Geometry: final body of the model. Coordinates: model frame, mm. A direction names the side the tool comes from. Coordinates: 2 decimals unless noted, no trailing zeros. Write each loop counter-clockwise with the first axis right and the second up, starting at its lowest first coordinate (ties: lowest second). Pieces come first, ordered by that corner, then holes. Notation, with made-up numbers: (1.25, 10.25) - (23.25, 10.25) arc R36 ccw to (23.25, 49.25) - close; hole circle Ø10 at (28.25, 26). An arc over 180 degrees is marked (long way). Put each result on its own line as item: value.
```python
from build123d import *

# Parameters (mm, degrees)
SKETCH1_W           = 419.1
SKETCH1_H           = 333.375
BOSS_EXTRUDE1_DEPTH = 107.95
SKETCH2_W           = 139.7
SKETCH2_H           = 50.8
CUT_EXTRUDE1_DEPTH  = 108.95
CHAMFER1_SIZE       = 50.8
CHAMFER1_SIZE2      = 13.611818976
FILLET1_R           = 12.7
SKETCH3_W           = 139.7
SKETCH3_H           = 56.403006085
CUT_EXTRUDE2_DEPTH  = 38.1
SKETCH4_W           = 139.7
SKETCH4_H           = 56.128435861
CUT_EXTRUDE3_DEPTH  = 38.1


with BuildPart() as part:
    # Sketch1 → Boss-Extrude1 (new body)
    with BuildSketch(Plane(origin=(0, 0, 0), x_dir=(1, 0, 0), z_dir=(0, 1, 0))):
        Rectangle(SKETCH1_W, SKETCH1_H)
    extrude(amount=BOSS_EXTRUDE1_DEPTH)

    # Sketch2 → Cut-Extrude1 (cut, through all)
    with BuildSketch(Plane(origin=(0, 107.95, 0), x_dir=(1, 0, 0), z_dir=(0, 1, 0))):
        with Locations((0, -115.8875)):
            Rectangle(SKETCH2_W, SKETCH2_H)
        Polygon((-69.85, -166.6875), (-69.85, -157.1625), (-32.169017961, -166.6875), align=None)
        Polygon((32.169017961, -166.6875), (69.85, -166.6875), (69.85, -157.1625), align=None)
    extrude(amount=-CUT_EXTRUDE1_DEPTH, mode=Mode.SUBTRACT)

    # Chamfer1
    chamfer1_edges = [part.edges().sort_by_distance(p)[0] for p in [
        (69.85, 53.975, 141.2875),
        (-69.85, 53.975, 141.2875),
    ]]
    chamfer1_side = [part.faces().sort_by_distance(p)[0] for p in [
        (0, 53.975, 141.2875),
    ]]
    chamfer(chamfer1_edges, length=CHAMFER1_SIZE, length2=CHAMFER1_SIZE2, reference=chamfer1_side[0])

    # Fillet1
    fillet1_edges = [part.edges().sort_by_distance(p)[0] for p in [
        (69.85, 53.975, 90.4875),
        (-69.85, 53.975, 90.4875),
        (-32.169017961, 53.975, 166.6875),
        (32.169017961, 53.975, 166.6875),
        (69.85, 53.975, 127.675681024),
        (-19.05, 53.975, 141.2875),
        (19.05, 53.975, 141.2875),
        (-69.85, 53.975, 127.675681024),
    ]]
    fillet(fillet1_edges, radius=FILLET1_R)

    # Sketch3 → Cut-Extrude2 (cut)
    with BuildSketch(Plane(origin=(0, 107.95, 0), x_dir=(1, 0, 0), z_dir=(0, 1, 0))):
        with Locations((0, -138.485996957)):
            Rectangle(SKETCH3_W, SKETCH3_H)
    extrude(amount=-CUT_EXTRUDE2_DEPTH, mode=Mode.SUBTRACT)

    # Sketch4 → Cut-Extrude3 (cut)
    with BuildSketch(Plane.XZ):
        with Locations((0, 138.623282069)):
            Rectangle(SKETCH4_W, SKETCH4_H)
    extrude(amount=-CUT_EXTRUDE3_DEPTH, mode=Mode.SUBTRACT)


solid = part.part
```
1. Section query C-C (x = -46.5). Return loops of the section in (y, z).
Answer below:
outline: (0, -166.69) - (107.95, -166.69) - (107.95, 90.49) - (0, 90.49) - close; (38.1, 133.93) - (69.85, 133.93) - (69.85, 163.06) - (38.1, 163.06) - close
2. Section query B-B (z = 113). Return loops of the section in (x, y), then the cut area to 3 significant figures.
Answer below:
outline: (-209.55, 0) - (-69.85, 0) - (-69.85, 107.95) - (-209.55, 107.95) - close; (69.85, 0) - (209.55, 0) - (209.55, 107.95) - (69.85, 107.95) - close
area: 30,200 mm²
3. Section query A-A (y = 61). Return loops of the section in (x, z), then the cut area to 3 significant figures.
Answer below:
outline: (-209.55, -166.69) - (209.55, -166.69) - (209.55, 166.69) - (69.85, 166.69) - (69.85, 157.16) - (33.7, 166.3) arc R12.7 ccw to (30.59, 166.69) - (-30.59, 166.69) arc R12.7 ccw to (-33.7, 166.3) - (-69.85, 157.16) - (-69.85, 166.69) - (-209.55, 166.69) - close; hole (-69.85, 103.19) arc R12.7 ccw to (-57.15, 90.49) - (57.15, 90.49) arc R12.7 ccw to (69.85, 103.19) - (69.85, 117.93) arc R12.7 ccw to (60.44, 130.2) - (20.67, 140.85) arc R12.7 ccw to (17.38, 141.29) - (-17.38, 141.29) arc R12.7 ccw to (-20.67, 140.85) - (-60.44, 130.2) arc R12.7 ccw to (-69.85, 117.93) - close
area: 133,000 mm²
4. Pin query (flat end, axial travel): pin 1 Ø24.5 at (x, z) = (-23.5, 149.5) entering from +Y. Return the tip coordinate at first contact, or that it passes through.
Answer below:
pin 1: stops at y = 69.85
5. Ray query, probe 1 along X at (y, z) = (8, 104); probe 2 along Z at (x, y) = (25.5, 44.5); probe 3 along Z at (x, y) = (-35.5, 93.5). Return the intervals inside material, ascending. Write a range as from..to.
Answer below:
probe 1: x = -209.55..-69.85, 69.85..209.55
probe 2: z = -166.69..90.49, 139.56..166.69
probe 3: z = -166.69..90.49
6. Mould query, pull axis X, two halves, no side actions, for faces 1 (the flat face through (-1, 55, 90.488)), 2 (the flat face through (-209.55, 53, 2)), 3 (the flat face through (139, 53, 166.688)). Classes: +X half, -X half, draft (parallel to the pull), parting line (faces both ways), or undercut.
Answer below:
face 1: undercut
face 2: -X half
face 3: draft
7. Set-up query: faces 4 (the flat face through (-52.029, 54.197, 161.667)), 5 (the cylindrical face through (-66.23, 53.22, 94.31)), 6 (the flat face through (-3, 0, -2)), 7 (the flat face through (-1, 38.1, 148)), 8 (the flat face through (0, 54, 166.688)). Return all of +Z, -Z, +X, -X, +Y, -Y with unobstructed straight access to the full face (end or side cutting, diameter ignored); none if empty.
Answer below:
face 4: +Z, +Y, -Y
face 5: +Y, -Y
face 6: +Z, -Z, +X, -X, -Y
face 7: +Z, -Y
face 8: +Z, +X, -X, +Y, -Y
8. Section query D-D (y = 90). Return loops of the section in (x, z).
Answer below:
outline: (-209.55, -166.69) - (209.55, -166.69) - (209.55, 166.69) - (69.85, 166.69) - (69.85, 103.19) arc R12.7 cw to (57.15, 90.49) - (-57.15, 90.49) arc R12.7 cw to (-69.85, 103.19) - (-69.85, 166.69) - (-209.55, 166.69) - close
